Verification items for this drawing (mm, ordinates from the low corner). A direction names the side the tool comes from. Coordinates: 2 decimals unless noted, no trailing zeros. Order: outer loops, then holes, each group sorted by start corner. A loop starts at its lowest first (then second) coordinate and runs counter-clockwise, first axis right, second up. Notation, with made-up numbers: (42, -38) -> (57, -38) arc R23 cw to (57, -30) -> close; hole circle Ø11 at (69, 61.5). An arc over 180 degrees is marked (long way). Answer in a Markdown table with one row per item. Add a question column.
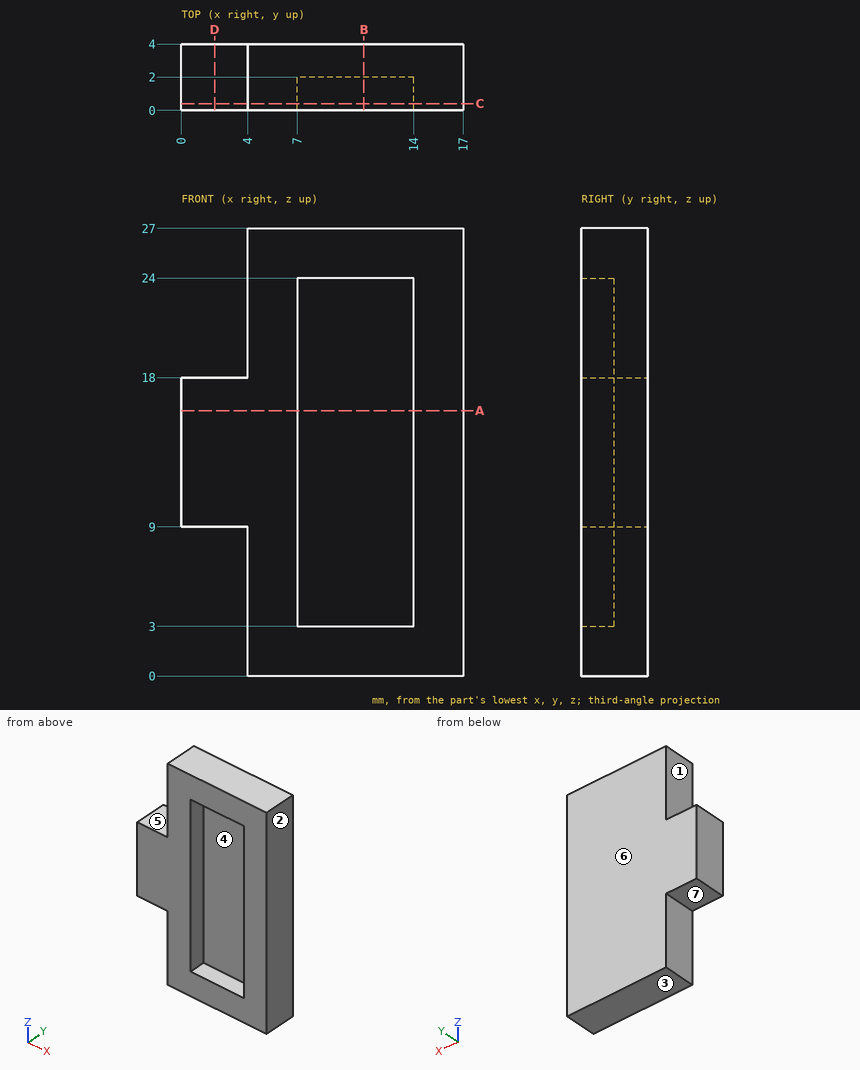
(1) Access from +Z, -Z, +X, -X, +Y, -Y to the whole of each face (thin tool, end or side, straight path). Record for the marked faces 5, 6 and 7.
(2) Mould release check, pull along X, two halves, no side actions. Record for the marked faces 1, 2, 3 and 4: +X half, -X half, draft (parallel to the pull), parting line (faces both ways), or undercut.
(3) Cross-section at C-C (y = 0.4). Enter the section's corners in (x, z).
(4) Cross-section at A-A (z = 16). Enter the section's corners in (x, y).
(5) Go/stop test with flat-tipped pins: P1, Ø2, axis at x = 2.5, y = 2.5, coming from the -Z side; P2, Ø3.5, axis at x = 10.5, z = 13.5, coming from the -Y side. Record where each tip stops, or that it passes through.
(6) Cross-section at B-B (x = 11). Enter the section's corners in (y, z).
(7) Cross-section at D-D (x = 2). Enter the section's corners in (y, z), plus the area to 3 significant figures.
(8) Scan lines: line 1 along X through (y, z) = (0.7, 10.5); line 2 along Z through (x, y) = (12, 1.5); line 3 along X through (y, z) = (0.3, 20.25). Record each from-to range of solid material in increasing order.
Checks:
| question | item | result |
|---|---|---|
| 1 | face 5 | +Z, -X, +Y, -Y |
| 1 | face 6 | +Z, -Z, +X, -X, +Y |
| 1 | face 7 | -Z, -X, +Y, -Y |
| 2 | face 1 | -X half |
| 2 | face 2 | +X half |
| 2 | face 3 | draft |
| 2 | face 4 | undercut |
| 3 | outline | (0, 9) -> (4, 9) -> (4, 0) -> (17, 0) -> (17, 27) -> (4, 27) -> (4, 18) -> (0, 18) -> close; hole (7, 3) -> (14, 3) -> (14, 24) -> (7, 24) -> close |
| 4 | outline | (0, 0) -> (7, 0) -> (7, 2) -> (14, 2) -> (14, 0) -> (17, 0) -> (17, 4) -> (0, 4) -> close |
| 5 | P1 | z = 9 |
| 5 | P2 | y = 2 |
| 6 | outline | (0, 0) -> (4, 0) -> (4, 27) -> (0, 27) -> (0, 24) -> (2, 24) -> (2, 3) -> (0, 3) -> close |
| 7 | outline | (0, 9) -> (4, 9) -> (4, 18) -> (0, 18) -> close |
| 7 | area | 36.0 mm² |
| 8 | line 1 | 0 to 7, 14 to 17 |
| 8 | line 2 | 0 to 3, 24 to 27 |
| 8 | line 3 | 4 to 7, 14 to 17 |
